Autodesk Inventor part; units mm, degrees
ref_plane "YZ Plane" through (0, 0, 0) normal (1, 0, 0) x (0, 1, 0)
ref_plane "XZ Plane" through (0, 0, 0) normal (0, 1, 0) x (-1, 0, 0)
ref_plane "XY Plane" through (0, 0, 0) normal (0, 0, 1) x (1, 0, 0)
sketch "Sketch2" plane through (0, 0, 0) normal (0, 0, 1) x (1, 0, 0)
  line L0 (0, 0) -> (44.45, 0)
  line L1 (44.45, 0) -> (44.45, 50.8)
  line L2 (44.45, 50.8) -> (0, 50.8)
  line L3 (0, 50.8) -> (0, 0)
  dimension "d0" = 50.8
  dimension "d1" = 44.45
extrude "Extrusion1" add sketch "Sketch2" along normal blind 25.4
sketch "Sketch3" plane through (0, 0, 25.4) normal (0, 0, 1) x (1, 0, 0)
  line L0 (2.54, 2.54) -> (20.32, 2.54)
  line L1 (20.32, 2.54) -> (20.32, 48.26)
  line L2 (20.32, 48.26) -> (2.54, 48.26)
  line L3 (2.54, 48.26) -> (2.54, 2.54)
  line L4 (0, 0) -> (44.45, 0)
  line L5 (0, 50.8) -> (0, 0)
  line L6 (44.45, 50.8) -> (0, 50.8)
  line L7 (21.59, 2.54) -> (41.91, 2.54)
  line L8 (41.91, 2.54) -> (41.91, 48.26)
  line L9 (41.91, 48.26) -> (21.59, 48.26)
  line L10 (21.59, 48.26) -> (21.59, 2.54)
  line L11 (44.45, 0) -> (44.45, 50.8)
  dimension "d4" = 2.54
  dimension "d5" = 2.54
  dimension "d6" = 2.54
  dimension "d7" = 20.32
  dimension "d8" = 2.54
  dimension "d9" = 2.54
  dimension "d10" = 2.54
  dimension "d11" = 22.86
extrude "Extrusion2" cut sketch "Sketch3" against normal blind 20.32 contours L3 L2 L1 L0 | L10 L9 L8 L7
sketch "Sketch4" plane through (0, 0, 0) normal (0, 0, -1) x (-1, 0, 0)
  circle A0 centre (-12.7, 17.78) radius 8.89
  line L0 (0, 50.8) -> (0, 0)
  line L1 (0, 0) -> (-44.45, 0)
  dimension "d14" = 17.78
  dimension "d17" = 12.7
  dimension "d18" = 17.78
extrude "Extrusion3" cut sketch "Sketch4" against normal blind 3.175
sketch "Sketch5" plane through (0, 0, 0) normal (0, 0, -1) x (-1, 0, 0)
  point P0 (0, 0)
sketch "Sketch6" plane through (12.7, 17.78, 3.175) normal (0, 0, -1) x (-1, 0, 0)
  circle A0 centre (0, 0) radius 8.89
  line L0 (0, 0) -> (-5.08, 0)
  line L1 (-5.08, 0) -> (-5.08, 12.7)
  line L2 (-5.08, 12.7) -> (0, 12.7)
  line L3 (0, 12.7) -> (0, 0)
  line L4 (0, 0) -> (5.08, 0)
  line L5 (5.08, 0) -> (5.08, 12.7)
  line L6 (5.08, 12.7) -> (0, 12.7)
  line L7 (0, 12.7) -> (0, 0)
  point P0 (12.7, -17.78)
  dimension "d21" = 12.7
  dimension "d22" = 5.08
  dimension "d23" = 5.08
extrude "Extrusion4" cut sketch "Sketch6" along normal blind 5.08 contours L5 L4 L3 A0 | A0 L3 L6 L5 | L1 L2 L3 A0 | A0 L3 L0 L1
sketch "Sketch7" plane through (0, 0, 3.175) normal (0, 0, -1) x (-1, 0, 0)
  point P0 (0, 0)
sketch "Sketch8" plane through (0, 0, 3.175) normal (0, 0, -1) x (-1, 0, 0)
  line L0 (-7.62, 25.0756) -> (-7.62, 30.48)
  line L1 (-17.78, 30.48) -> (-7.62, 30.48)
  line L2 (-7.62, 30.48) -> (-7.62, 26.67)
  line L3 (-7.62, 26.67) -> (-17.78, 26.67)
  line L4 (-17.78, 26.67) -> (-17.78, 30.48)
  point P0 (0, 0)
  dimension "d26" = 3.81
extrude "Extrusion5" cut sketch "Sketch8" against normal blind 2.54
sketch "Sketch14" plane through (41.91, 2.54, 25.4) normal (-1, 0, 0) x (0, 0, 1)
  line L0 (0, 0) -> (-20.32, 0)
  line L1 (0, 45.72) -> (-20.32, 45.72)
  line L2 (-12.7, 45.72) -> (-12.7, 43.18)
  line L3 (-12.7, 43.18) -> (-15.24, 45.72)
  line L4 (-12.7, 0) -> (-12.7, 2.54)
  line L5 (-12.7, 2.54) -> (-15.24, 0)
  point P0 (-25.4, -2.54)
  dimension "d52" = 45
  dimension "d53" = 2.54
  dimension "d54" = 2.54
  dimension "d55" = 45
  dimension "d56" = 5.08
  dimension "d57" = 5.08
extrude "Arduino Holder" add sketch "Sketch14" along normal blind 20.32
sketch "Sketch16" plane through (2.54, 2.54, 25.4) normal (0, 1, 0) x (1, 0, 0)
  line L0 (0, 12.7) -> (3.81, 12.7)
  line L1 (3.81, 12.7) -> (0, 16.51)
  line L2 (0, 0) -> (0, 20.32)
  line L3 (17.78, 5.08) -> (17.78, 20.32)
  line L4 (17.78, 16.51) -> (13.97, 12.7)
  line L5 (13.97, 12.7) -> (17.78, 12.7)
  line L6 (17.78, 20.32) -> (0, 20.32)
  point P0 (-2.54, 25.4)
  dimension "d60" = 45
  dimension "d61" = 3.81
  dimension "d62" = 3.81
  dimension "d64" = 45
  dimension "d144" = 7.62
  dimension "d145" = 7.62
extrude "Bluetooth Holder" add sketch "Sketch16" along normal blind 45.72
sketch "Sketch17" plane through (0, 0, 0) normal (-1, 0, 0) x (0, 0, 1)
  line L0 (0, 50.8) -> (25.4, 50.8)
  line L1 (0, 0) -> (5.08, 0)
  line L2 (5.08, 0) -> (5.08, 50.8)
  line L3 (5.08, 50.8) -> (0, 50.8)
  line L4 (0, 50.8) -> (0, 0)
  dimension "d68" = 5.08
extrude "Extrusion13" add sketch "Sketch17" along normal blind 5.08
sketch "Sketch18" plane through (0, 0, 5.08) normal (0, 0, 1) x (1, 0, 0)
  line L0 (0, 50.8) -> (0, 0)
  line L1 (0, 2.54) -> (-2.54, 2.54)
  line L2 (-2.54, 2.54) -> (-2.54, 48.26)
  line L3 (-2.54, 48.26) -> (0, 48.26)
  line L4 (0, 48.26) -> (0, 2.54)
  line L5 (0, 50.8) -> (-5.08, 50.8)
  line L6 (0, 0) -> (-5.08, 0)
  dimension "d71" = 2.54
  dimension "d72" = 2.54
  dimension "d73" = 2.54
extrude "Extrusion14" cut sketch "Sketch18" against normal blind 5.08
sketch "Sketch19" plane through (44.45, 0, 0) normal (1, 0, 0) x (0, 0, -1)
  line L0 (0, 50.8) -> (-25.4, 50.8)
  line L1 (0, 0) -> (-5.08, 0)
  line L2 (-5.08, 0) -> (-5.08, 50.8)
  line L3 (-5.08, 50.8) -> (0, 50.8)
  line L4 (0, 50.8) -> (0, 0)
  dimension "d76" = 5.08
extrude "Extrusion15" add sketch "Sketch19" along normal blind 5.08
sketch "Sketch21" plane through (44.45, 0, 5.08) normal (0, 0, 1) x (1, 0, 0)
  line L0 (0, 0) -> (0, 50.8)
  line L1 (0, 2.54) -> (2.54, 2.54)
  line L2 (2.54, 2.54) -> (2.54, 48.26)
  line L3 (2.54, 48.26) -> (0, 48.26)
  line L4 (0, 48.26) -> (0, 2.54)
  line L5 (0, 50.8) -> (5.08, 50.8)
  line L6 (0, 0) -> (5.08, 0)
  line L7 (5.08, 50.8) -> (5.08, 0)
  point P0 (-44.45, 0)
  dimension "d79" = 2.54
  dimension "d81" = 2.54
  dimension "d82" = 2.54
extrude "Extrusion16" cut sketch "Sketch21" against normal blind 5.08 contours L0 L3 L2 L1
sketch "Sketch28" plane through (0, 0, 25.4) normal (-1, 0, 0) x (0, 0, 1)
  line L0 (-20.32, 0) -> (0, 0)
  line L1 (0, 50.8) -> (-10.16, 50.8)
  line L2 (-10.16, 50.8) -> (-10.16, 0)
  line L3 (-10.16, 0) -> (0, 0)
  line L4 (0, 0) -> (0, 50.8)
  point P0 (-25.4, 0)
  dimension "d141" = 10.16
extrude "Height Reduce" cut sketch "Sketch28" against normal blind 48.26
sketch "Sketch30" plane through (0, 0, 5.08) normal (0, 0, 1) x (1, 0, 0)
  line L0 (22.86, 5.08) -> (40.64, 5.08)
  line L1 (40.64, 5.08) -> (40.64, 26.67)
  line L2 (40.64, 26.67) -> (22.86, 26.67)
  line L3 (22.86, 26.67) -> (22.86, 5.08)
  line L4 (21.59, 2.54) -> (21.59, 48.26)
  line L5 (41.91, 48.26) -> (41.91, 2.54)
  line L6 (41.91, 2.54) -> (21.59, 2.54)
  point P0 (0, 0)
  point P1 (24.13, 12.7)
  point P2 (44.45, 30.48)
  dimension "d146" = 1.27
  dimension "d147" = 1.27
  dimension "d148" = 21.59
  dimension "d149" = 2.54
  dimension "d150" = 17.78
extrude "Extrusion27" cut sketch "Sketch30" against normal blind 2.54
sketch "Sketch31" plane through (0, 0, 5.08) normal (0, 0, 1) x (1, 0, 0)
  line L0 (21.59, 2.54) -> (21.59, 48.26)
  line L1 (41.91, 48.26) -> (41.91, 2.54)
  line L2 (21.59, 45.72) -> (41.91, 45.72)
  line L3 (41.91, 45.72) -> (41.91, 29.21)
  line L4 (41.91, 29.21) -> (21.59, 29.21)
  line L5 (21.59, 29.21) -> (21.59, 45.72)
  line L6 (21.59, 48.26) -> (41.91, 48.26)
  line L7 (21.59, 41.275) -> (30.48, 41.275)
  line L8 (30.48, 41.275) -> (30.48, 33.655)
  line L9 (30.48, 33.655) -> (21.59, 33.655)
  line L10 (21.59, 33.655) -> (21.59, 41.275)
  line L11 (41.91, 45.72) -> (36.83, 45.72)
  line L12 (36.83, 45.72) -> (36.83, 29.21)
  line L13 (36.83, 29.21) -> (41.91, 29.21)
  line L14 (41.91, 29.21) -> (41.91, 45.72)
  point P0 (0, 0)
  point P1 (24.13, 33.02)
  dimension "d157" = 2.54
  dimension "d158" = 16.51
  dimension "d159" = 4.445
  dimension "d160" = 7.62
  dimension "d161" = 8.89
  dimension "d162" = 4.445
  dimension "d163" = 5.08
extrude "Extrusion28" cut sketch "Sketch31" against normal blind 25.4 contours L0 L7 L8 L9
extrude "Extrusion29" cut sketch "Sketch31" against normal blind 2.54 contours L12 L2 L1 L4
extrude "Extrusion30" cut sketch "Sketch31" against normal blind 1.27 contours L0 L9 L8 L7 L2 L12 L4
sketch "Sketch33" plane through (44.45, 2.54, 0) normal (1, 0, 0) x (0, 0, -1)
  line L0 (-5.08, 48.26) -> (-15.24, 48.26)
  line L1 (-15.24, -2.54) -> (-12.7, -2.54)
  line L2 (-12.7, -2.54) -> (-12.7, 48.26)
  line L3 (-12.7, 48.26) -> (-15.24, 48.26)
  line L4 (-15.24, 48.26) -> (-15.24, -2.54)
  point P0 (0, -2.54)
  dimension "d194" = 2.54
extrude "Extrusion33" add sketch "Sketch33" along normal blind 2.54
sketch "Sketch35" plane through (0, 2.54, 0) normal (-1, 0, 0) x (0, 0, 1)
  line L0 (5.08, 48.26) -> (15.24, 48.26)
  line L1 (15.24, -2.54) -> (12.7, -2.54)
  line L2 (12.7, -2.54) -> (12.7, 48.26)
  line L3 (12.7, 48.26) -> (15.24, 48.26)
  line L4 (15.24, 48.26) -> (15.24, -2.54)
  point P0 (0, -2.54)
  dimension "d197" = 2.54
extrude "Extrusion34" add sketch "Sketch35" along normal blind 2.54
sketch "Sketch36" plane through (-5.08, 0, 5.08) normal (0, -1, 0) x (1, 0, 0)
  line L0 (2.54, 10.16) -> (5.08, 7.62)
  line L1 (5.08, 7.62) -> (2.54, 7.62)
  line L2 (5.08, 7.62) -> (2.54, 7.62)
  line L3 (2.54, 7.62) -> (2.54, 10.16)
  line L4 (49.53, 7.62) -> (52.07, 10.16)
  line L5 (52.07, 10.16) -> (52.07, 7.62)
  line L6 (52.07, 7.62) -> (49.53, 7.62)
  point P0 (5.08, -5.08)
extrude "Extrusion35" cut sketch "Sketch36" against normal blind 50.8
sketch "Sketch37" plane through (-5.08, 50.8, 5.08) normal (0, 1, 0) x (1, 0, 0)
  line L0 (52.07, -10.16) -> (2.54, -10.16)
  line L1 (43.18, -10.16) -> (30.48, -10.16)
  line L2 (30.48, -10.16) -> (30.48, -7.62)
  line L3 (30.48, -7.62) -> (43.18, -7.62)
  line L4 (43.18, -7.62) -> (43.18, -10.16)
  line L5 (26.67, -10.16) -> (26.67, -7.62)
  line L6 (46.99, -10.16) -> (46.99, -7.62)
  point P0 (5.08, 5.08)
  dimension "d202" = 2.54
  dimension "d203" = 12.7
  dimension "d204" = 3.81
  dimension "d205" = 3.81
extrude "USB hole" cut sketch "Sketch37" against normal blind 2.54
sketch "Sketch38" plane through (20.32, 2.54, 5.08) normal (-1, 0, 0) x (0, 0, 1)
  line L0 (0, 0) -> (3.81, 3.81)
  line L1 (3.81, 3.81) -> (3.81, 41.91)
  line L2 (3.81, 41.91) -> (0, 45.72)
  line L3 (0, 45.72) -> (0, 0)
  line L4 (3.81, 3.81) -> (10.16, 3.81)
  line L5 (10.16, 3.81) -> (10.16, 41.91)
  line L6 (10.16, 0) -> (10.16, 45.72)
  line L7 (10.16, 41.91) -> (3.81, 41.91)
  point P0 (-5.08, -2.54)
  dimension "d209" = 3.81
  dimension "d210" = 135
  dimension "d211" = 135
extrude "Center column remove" cut sketch "Sketch38" along normal mid plane 7.62
properties part number "nano_enclosure_v3"
For this review, take the finished solid that the model builds, in its own axes (mm). A direction names the side the tool comes from. Give positions to 0.01 mm unless a question says otherwise; leave off trailing zeros. Order: outer loops, then holes, each group sorted by start corner. A loop starts at its lowest first (then second) coordinate and runs counter-clockwise, first axis right, second up. Notation, with made-up numbers: (-35, 26) - (-28, 26) arc R22 cw to (-28, 36) - close; hole circle Ø2 at (83, 88). An arc over 180 degrees is marked (long way). Answer as a JSON object with one key per item and string values. Group by question number.
Item 1: Wall thickness on line 1 along X through (y, z) = (17.78, 1.6); line 2 along X through (y, z) = (45.5, 3.25); line 3 along Y through (x, z) = (15.5, 12.5): over which ranges is each line inside the solid? List them lowest first.
Item 2: Take a section at B-B on x = 12.7. Give the boundary of the cut face in (y, z) (3 decimals).
Item 3: Take a section at C-C on z = 1.75. Give the boundary of the cut face in (x, y) (3 decimals), and give its area (3 significant figures).
Item 4: Machinability: for faces 3 (the flat face through (4.47, 25.08, 10.82)), 4 (the flat face through (25.4, 50, 14)), 5 (the cylindrical face through (13.015, 8.896, 1.565)), 6 (the flat face through (32, 4, 12.7)), which of the approach directions +Z, -Z, +X, -X, +Y, -Y give a long, thin tool a straight path to every point of the face, cutting with its end or side? Answer none if there is none.
Item 5: Draft analysis for pull direction X (two halves, no side actions). For faces 1 (the flat face through (13, 26.67, 4)), 2 (the flat face through (-4, 25, 5.08)), state which applies: pulls with the +X half, pulls with the -X half, needs draft (parallel to the pull), parting line crosses it, or undercut.
Item 6: Clearance check with flat-ended pins moving along their axes: pin 1 Ø1.5 at (x, y) = (23, 8) entering from +Z; pin 2 Ø8 at (y, z) = (45, 10) entering from -X; pin 3 Ø12 at (x, y) = (32.5, 15) entering from +Z. State where each tip first meets the part, or that it passes through.
Item 7: Take a section at A-A on y = 17.78. Give the number of separate pieces and of enclosed holes in the cut face, and give its area (3 significant figures).
Item 8: Take a section at D-D on y = 35.5. Give the boundary of the cut face in (x, z).
Reported:
{
 "1": {"line 1": "-5.08 to -2.54, 0 to 3.81, 21.59 to 44.45, 46.99 to 49.53", "line 2": "-5.08 to -2.54, 0 to 36.83, 41.91 to 44.45, 46.99 to 49.53", "line 3": "0 to 2.54, 48.26 to 50.8"},
 "2": {"outline": "(0, 0) - (8.89, 0) - (8.89, 3.175) - (26.67, 3.175) - (26.67, 5.08) - (2.54, 5.08) - (2.54, 15.24) - (0, 15.24) - close; (30.48, 0) - (50.8, 0) - (50.8, 15.24) - (48.26, 15.24) - (48.26, 5.08) - (30.48, 5.08) - close"},
 "3": {"outline": "(-5.08, 0) - (49.53, 0) - (49.53, 50.8) - (-5.08, 50.8) - close; hole (-2.54, 2.54) - (0, 2.54) - (0, 48.26) - (-2.54, 48.26) - close; hole (7.62, 25.076) arc R8.89 ccw (long way) to (17.78, 25.076) - (17.78, 30.48) - (7.62, 30.48) - close; hole (21.59, 33.655) - (30.48, 33.655) - (30.48, 41.275) - (21.59, 41.275) - close; hole (44.45, 2.54) - (46.99, 2.54) - (46.99, 48.26) - (44.45, 48.26) - close", "area": "2,180 mm^2"},
 "4": {"face 3": "none", "face 4": "+Z, +Y", "face 5": "-Z", "face 6": "+Z"},
 "5": {"face 1": "undercut", "face 2": "needs draft"},
 "6": {"pin 1": "z = 5.08", "pin 2": "x = -1.3", "pin 3": "z = 2.54"},
 "7": {"separate pieces": "3", "enclosed holes": "0", "area": "215 mm^2"},
 "8": {"outline": "(-5.08, 0) - (-2.54, 0) - (-2.54, 5.08) - (-5.08, 5.08) - close; (-2.54, 15.24) - (0, 12.7) - (0, 0) - (21.59, 0) - (21.59, 5.08) - (2.54, 5.08) - (2.54, 8.89) - (6.35, 12.7) - (2.54, 12.7) - (2.54, 15.24) - close; (30.48, 0) - (44.45, 0) - (44.45, 12.7) - (46.99, 15.24) - (41.91, 15.24) - (41.91, 2.54) - (36.83, 2.54) - (36.83, 3.81) - (30.48, 3.81) - close; (46.99, 0) - (49.53, 0) - (49.53, 5.08) - (46.99, 5.08) - close"}
}
